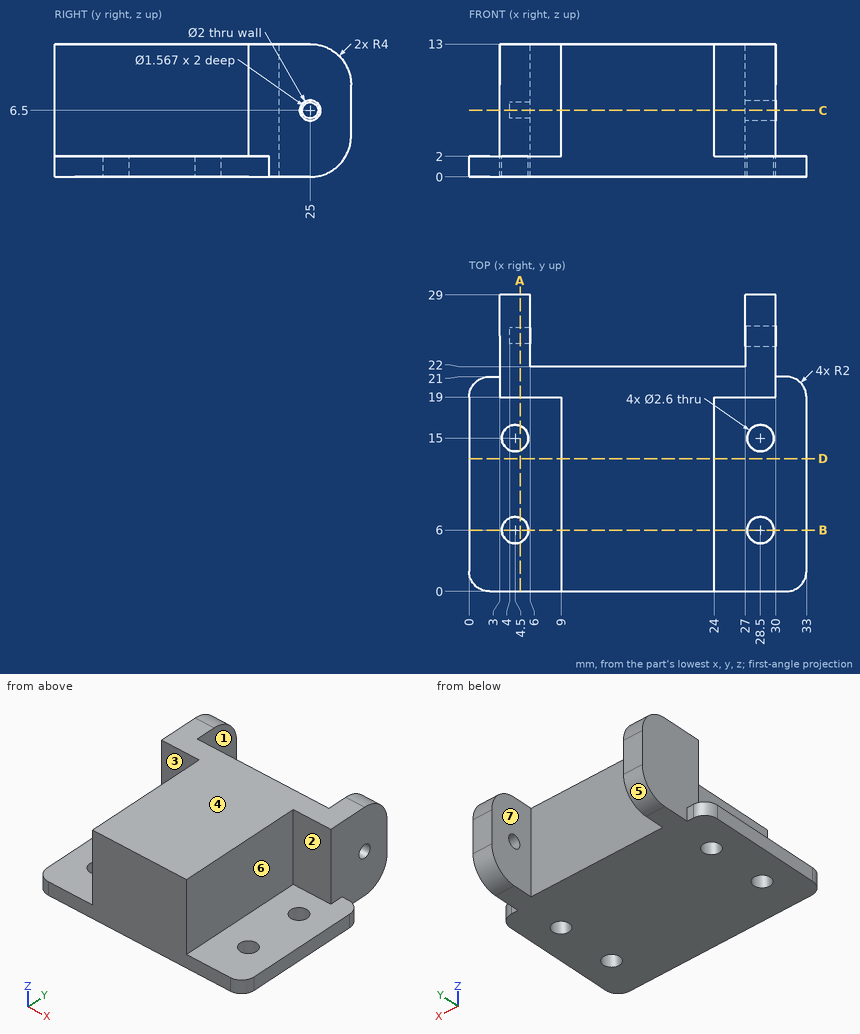
Design review of the part shown in the three views and the two pictorial views. Dimensions are in mm from the part's minimum x, y and z. A direction names the side the tool comes from. Give positions to 0.01 mm unless a question says otherwise; leave off trailing zeros. Write each loop counter-clockwise with the first axis right and the second up, starting at its lowest first coordinate (ties: lowest second). Pieces come first, ordered by that corner, then holes. Notation, with made-up numbers: M 39.5,17 L 96.5,17 A19 ccw 96.5,41 Z; hole C 5.25,34 d5. An arc over 180 degrees is marked long. Answer in a Markdown table with one row per item.
Item 1: Add section D-D on y = 13. Give the boundary of the cut face in (x, z), plus the area to 3 significant figures.
Check sheet entries:
| item | result |
|---|---|
| outline | M 0,0 L 33,0 L 33,2 L 24,2 L 24,13 L 9,13 L 9,2 L 0,2 Z |
| area | 231 mm2 |
Item 2: For line 1 along X through (y, z) = (6, 1); line 2 along Y through (x, z) = (5.55, 6.5); line 3 along Y through (x, z) = (28.2, 6.5), list the stretches that pass through material, from the lowest coordinate up.
Check sheet entries:
| item | result |
|---|---|
| line 1 | 0 to 3.2, 5.8 to 27.2, 29.8 to 33 |
| line 2 | 19 to 24.22, 25.78 to 29 |
| line 3 | 19 to 24, 26 to 29 |
Item 3: Draft analysis for pull direction X (two halves, no side actions). For the marked faces 5, 6 and 7, state which applies: +X half, -X half, draft (parallel to the pull), parting line (faces both ways), or undercut.
Check sheet entries:
| item | result |
|---|---|
| face 5 | draft |
| face 6 | +X half |
| face 7 | undercut |
Item 4: Tool access review of the marked faces 1, 2, 3 and 4: name each direction out of +Z, -Z, +X, -X, +Y, -Y from which nothing blocks a thin tool from reaching the whole face with its end or side.
Check sheet entries:
| item | result |
|---|---|
| face 1 | +Z, -Z, +Y |
| face 2 | +Z, +X, -Y |
| face 3 | +Z, -X, -Y |
| face 4 | +Z, +X, -X, +Y, -Y |
Item 5: Add section C-C on z = 6.5. Give the boundary of the cut face in (x, y).
Check sheet entries:
| item | result |
|---|---|
| outline | M 3,19 L 9,19 L 9,0 L 24,0 L 24,19 L 30,19 L 30,24 L 27,24 L 27,22 L 6,22 L 6,24.22 L 4,24.22 L 4,25.78 L 6,25.78 L 6,29 L 3,29 Z; M 27,26 L 30,26 L 30,29 L 27,29 Z |
Item 6: Add section B-B on y = 6. Give the boundary of the cut face in (x, z), plus the area to 3 significant figures.
Check sheet entries:
| item | result |
|---|---|
| outline | M 0,0 L 3.2,0 L 3.2,2 L 0,2 Z; M 5.8,0 L 27.2,0 L 27.2,2 L 24,2 L 24,13 L 9,13 L 9,2 L 5.8,2 Z; M 29.8,0 L 33,0 L 33,2 L 29.8,2 Z |
| area | 221 mm2 |
Item 7: For P1, Ø2.5, axis at y = 25, z = 6.5, coming from the -X side; P2, Ø2, axis at x = 13.5, z = 2.5, coming from the +Y side; P3, Ø0.5, axis at x = 2.5, z = 1, coming from the +Y side, all flat-tipped, find the tip position at first contact; note any pin that passes through.
Check sheet entries:
| item | result |
|---|---|
| P1 | x = 3 |
| P2 | y = 22 |
| P3 | y = 21 |
Item 8: Add section A-A on x = 5. Give the boundary of the cut face in (y, z), plus the area to 3 significant figures.
Check sheet entries:
| item | result |
|---|---|
| outline | M 0,0 L 4.8,0 L 4.8,2 L 0,2 Z; M 7.2,0 L 13.8,0 L 13.8,2 L 7.2,2 Z; M 16.2,0 L 25,0 A4 ccw 29,4 L 29,9 A4 ccw 25,13 L 19,13 L 19,2 L 16.2,2 Z; hole C 25,6.5 d1.57 |
| area | 150 mm2 |
